Part model, mm, in its own coordinate system. Face numbers are marked on the shaded views. Round coordinates to 2 decimals unless told otherwise and drop trailing zeros. Order: outer loops, then holes, each group sorted by start corner. A loop starts at its lowest first (then second) coordinate and runs counter-clockwise, first axis right, second up. Notation, with made-up numbers: (-17.75, -25) -> (28.25, -25) arc R26 cw to (28.25, 3) -> close; hole circle Ø9 at (73.5, 10.5). An arc over 180 degrees is marked (long way). Answer as a JSON object with one key per item and string values. Group by question number.
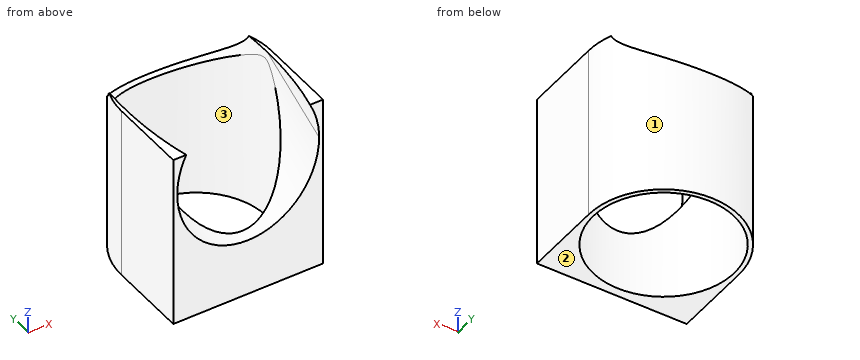
```python
from build123d import *

# Parameters (mm, degrees)
SKETCH1_R           = 17.15
SKETCH1_R_2         = 16.15
BOSS_EXTRUDE1_DEPTH = 40
BOSS_EXTRUDE3_DEPTH = 40
SKETCH2_R           = 16.25
CUT_EXTRUDE1_DEPTH  = 302.327569717


with BuildPart() as part:
    # Sketch1 → Boss-Extrude1 (new body)
    with BuildSketch(Plane.XY):
        with Locations((0, 200)):
            Circle(SKETCH1_R)
        with Locations((0, 200)):
            Circle(SKETCH1_R_2, mode=Mode.SUBTRACT)
    extrude(amount=-BOSS_EXTRUDE1_DEPTH)

    # Sketch4 → Boss-Extrude3 (add)
    with BuildSketch(Plane(origin=(0, 0, -40), x_dir=(-1, 0, 0), z_dir=(0, 0, -1))):
        Polygon((17.15, 182.85), (17.15, 181.85), (-17.15, 181.85), (-17.15, 182.85), (0, 182.85), align=None)
        with BuildLine():
            Line((17.15, 182.85), (17.15, 200))
            ThreePointArc((17.15, 200), (12.126881297, 187.873118703), (0, 182.85))
            Line((0, 182.85), (17.15, 182.85))
        make_face()
        with BuildLine():
            ThreePointArc((0, 182.85), (-12.126881297, 187.873118703), (-17.15, 200))
            Line((-17.15, 200), (-17.15, 182.85))
            Line((-17.15, 182.85), (0, 182.85))
        make_face()
    extrude(amount=-BOSS_EXTRUDE3_DEPTH)

    # Sketch2 → Cut-Extrude1 (cut, through all)
    with BuildSketch(Plane(origin=(0, 401.975230219, 196.056419574), x_dir=(1, 0, 0), z_dir=(0, 0.898794046, 0.438371147))):
        with Locations((0, 87.674229358)):
            Circle(SKETCH2_R)
    extrude(amount=-CUT_EXTRUDE1_DEPTH, mode=Mode.SUBTRACT)


solid = part.part
```
Q1. Band-saw the part on C-C (x = 0). List the corners of the cut face in (y, z), plus the area to 3 significant figures.
Q2. Drop flat-ended pins along their axis: pin 1 Ø10 at (y, z) = (211.5, -31) entering from -X; pin 2 Ø6 at (y, z) = (209.5, -9.5) entering from +X. Give the stop position or say it passes through.
Q3. Two-plate mould, pull along X, no slides. Class the marked faces 1, 2 and 3: +X half, -X half, draft (parallel to the pull), parting line (faces both ways), or undercut.
Q4. Band-saw the part on A-A (x = 5.5). List the corners of the cut face in (y, z), plus the area to 3 significant figures.
Q5. Band-saw the part on B-B (z = -28.5). List the corners of the cut face in (x, y), plus the area to 3 significant figures.
Q6. Wall check: line 1 (X direction, y = 200, z = -14.5); line 2 (Y direction, x = -9, z = -36.5); line 3 (Y direction, x = -9.5, z = -21.5). Give the ranges that are in metal, low to high. Write a range as [from, to].
Completed:
{
 "1": {"outline": "(181.85, -40) -> (183.85, -40) -> (183.85, -25.96) -> (181.85, -26.93) -> close; (216.15, -40) -> (217.15, -40) -> (217.15, -9.72) -> (216.15, -10.2) -> close", "area": "57.2 mm2"},
 "2": {"pin 1": "x = -15.87", "pin 2": "x = 15.87"},
 "3": {"face 1": "parting line", "face 2": "draft", "face 3": "undercut"},
 "4": {"outline": "(181.85, -40) -> (184.82, -40) -> (184.82, -24.42) -> (181.85, -25.87) -> close; (215.18, -40) -> (216.24, -40) -> (216.24, -9.09) -> (215.18, -9.61) -> close", "area": "76.5 mm2"},
 "5": {"outline": "(-17.15, 181.85) -> (17.15, 181.85) -> (17.15, 200) arc R17.15 ccw to (-17.15, 200) -> close; hole circle Ø32.3 at (0, 200)", "area": "265 mm2"},
 "6": {"line 1": "[-17.15, -16.15], [16.15, 17.15]", "line 2": "[181.85, 186.59], [213.41, 214.6]", "line 3": "[185.99, 186.94], [213.06, 214.28]"}
}
